from build123d import *

# Parameters (mm, degrees)
SKETCH1_R           = 27.305
BOSS_EXTRUDE1_DEPTH = 2.54
SKETCH2_R           = 25.4
BOSS_EXTRUDE2_DEPTH = 2.54
CUT_EXTRUDE1_REACH  = 7.08
SKETCH3_R           = 3.334616924
SKETCH3_R_2         = 2.413


with BuildPart() as part:
    # Sketch1 → Boss-Extrude1 (new body)
    with BuildSketch(Plane(origin=(0, 0, 0), x_dir=(1, 0, 0), z_dir=(0, 1, 0))):
        Circle(SKETCH1_R)
    extrude(amount=BOSS_EXTRUDE1_DEPTH)

    # Sketch2 → Boss-Extrude2 (add)
    with BuildSketch(Plane(origin=(0, 2.54, 0), x_dir=(1, 0, 0), z_dir=(0, 1, 0))):
        Circle(SKETCH2_R)
    extrude(amount=BOSS_EXTRUDE2_DEPTH)

    # Sketch3 → Cut-Extrude1 (cut, up to next)
    with BuildSketch(Plane.XZ, mode=Mode.PRIVATE) as cut_extrude1_sk1:
        Circle(SKETCH3_R)
    cut_extrude1_tool1 = extrude(cut_extrude1_sk1.sketch, amount=-CUT_EXTRUDE1_REACH, mode=Mode.PRIVATE) & part.part
    add(cut_extrude1_tool1.solids().sort_by_distance((0, 0, 0))[0], mode=Mode.SUBTRACT)
    # Sketch3 → Cut-Extrude1 (cut, up to next)
    with BuildSketch(Plane.XZ, mode=Mode.PRIVATE) as cut_extrude1_sk2:
        with Locations((-19.05, 0)):
            Circle(SKETCH3_R_2)
    cut_extrude1_tool2 = extrude(cut_extrude1_sk2.sketch, amount=-CUT_EXTRUDE1_REACH, mode=Mode.PRIVATE) & part.part
    add(cut_extrude1_tool2.solids().sort_by_distance((-19.05, 0, 0))[0], mode=Mode.SUBTRACT)
    # Sketch3 → Cut-Extrude1 (cut, up to next)
    with BuildSketch(Plane.XZ, mode=Mode.PRIVATE) as cut_extrude1_sk3:
        with Locations((19.05, 0)):
            Circle(SKETCH3_R_2)
    cut_extrude1_tool3 = extrude(cut_extrude1_sk3.sketch, amount=-CUT_EXTRUDE1_REACH, mode=Mode.PRIVATE) & part.part
    add(cut_extrude1_tool3.solids().sort_by_distance((19.05, 0, 0))[0], mode=Mode.SUBTRACT)


solid = part.part
Can you work these out from the model? Positions are in its coordinate system, mm. A direction names the side the tool comes from. Coordinates: 2 decimals unless noted, no trailing zeros. Write each loop counter-clockwise with the first axis right and the second up, starting at its lowest first coordinate (ties: lowest second). Pieces come first, ordered by that corner, then holes. Notation, with made-up numbers: (1.5, 82.5) -> (24.5, 82.5) arc R32 ccw to (24.5, 109.5) -> close; hole circle Ø4 at (14, -6.5). An arc over 180 degrees is marked (long way). Write item = value, one per line.
(1) Imagine slicing it at D-D (x = -20). Please give me the cut outline in (y, z).
Verdict:
outline = (0, -18.59) -> (2.54, -18.59) -> (2.54, -15.66) -> (5.08, -15.66) -> (5.08, -2.22) -> (0, -2.22) -> close; (0, 2.22) -> (5.08, 2.22) -> (5.08, 15.66) -> (2.54, 15.66) -> (2.54, 18.59) -> (0, 18.59) -> close
(2) For pin 1 (3 mm diameter, centred on y = 1, z = 4.5, fed in from +X); pin 2 (4 mm diameter, centred on x = 0, z = 0, fed in from +Y); pin 3 (2 mm diameter, centred on x = 2.5, y = 1.5, fed in from -Z); pin 4 (3 mm diameter, centred on y = 3, z = 10.5, fed in from -X), each with a flat end and sliding along its axis, tell me the tip position at first contact or that it passes through.
Verdict:
pin_1 = 27.14
pin_2 = through
pin_3 = -27.26
pin_4 = -25.75
(3) Imagine slicing it at B-B (z = 0). Please give me the cut outline in (x, y) (3 decimals), and give its area (3 significant figures).
Verdict:
outline = (-27.305, 0) -> (-21.463, 0) -> (-21.463, 5.08) -> (-25.4, 5.08) -> (-25.4, 2.54) -> (-27.305, 2.54) -> close; (-16.637, 0) -> (-3.335, 0) -> (-3.335, 5.08) -> (-16.637, 5.08) -> close; (3.335, 0) -> (16.637, 0) -> (16.637, 5.08) -> (3.335, 5.08) -> close; (21.463, 0) -> (27.305, 0) -> (27.305, 2.54) -> (25.4, 2.54) -> (25.4, 5.08) -> (21.463, 5.08) -> close
area = 185 mm^2
(4) Imagine slicing it at C-C (y = 0.7). Please give me the cut outline in (x, z) (3 decimals), and give its area (3 significant figures).
Verdict:
outline = circle Ø54.61 at (0, 0); hole circle Ø4.826 at (-19.05, 0); hole circle Ø6.669 at (0, 0); hole circle Ø4.826 at (19.05, 0)
area = 2,270 mm^2
(5) Thinking about a two-plate mould opening in X: for faces 3 (the face through (6, 0, 0)), 4 (the face through (-3.555, 1.252, -27.073)), 5 (the face through (3.18, 2.5, 1)), 6 (the face through (-16.748, 2.504, 0.725)), which applies, +X half, -X half, draft (parallel to the pull), parting line (faces both ways), or undercut?
Verdict:
face_3 = draft
face_4 = parting line
face_5 = undercut
face_6 = undercut
(6) If I drill on probe 1 along X at (y, z) = (3.4, 1); probe 2 along Z at (x, y) = (0, 4); probe 3 along Z at (x, y) = (20.5, 3.85), over which ranges is the centre line in solid material (lowest first)?
Verdict:
probe_1 = -25.38 to -21.25, -16.85 to -3.18, 3.18 to 16.85, 21.25 to 25.38
probe_2 = -25.4 to -3.33, 3.33 to 25.4
probe_3 = -15 to -1.93, 1.93 to 15
(7) On a 3-axis mill with a long thin cutter (end or side, diameter ignored), from which of +Z, -Z, +X, -X, +Y, -Y can I reach the whole of each face in a straight line? I mean faces 1 (the face through (18.1, 2.54, 18.1)), 2 (the face through (16.64, 2.5, 0.11)). Say none if no direction works.
Verdict:
face_1 = +Y
face_2 = +Y, -Y
(8) Imagine slicing it at A-A (x = 0). Please give me the cut outline in (y, z) (3 decimals), and give its area (3 significant figures).
Verdict:
outline = (0, -27.305) -> (2.54, -27.305) -> (2.54, -25.4) -> (5.08, -25.4) -> (5.08, -3.335) -> (0, -3.335) -> close; (0, 3.335) -> (5.08, 3.335) -> (5.08, 25.4) -> (2.54, 25.4) -> (2.54, 27.305) -> (0, 27.305) -> close
area = 234 mm^2
